Model file for the job. Use its own axes, mm. Give positions to 0.01 mm unless a question says otherwise; leave off trailing zeros. Write each loop counter-clockwise with the first axis right and the second up, starting at its lowest first coordinate (ties: lowest second). Pieces come first, ordered by that corner, then holes. Notation, with made-up numbers: (68, -10.5) - (72, -10.5) arc R5 ccw to (72, -5.5) - close; hole circle Ø4 at (-31, 55). An arc over 180 degrees is marked (long way). Use CSV: the item, a comma, the result in double quotes.
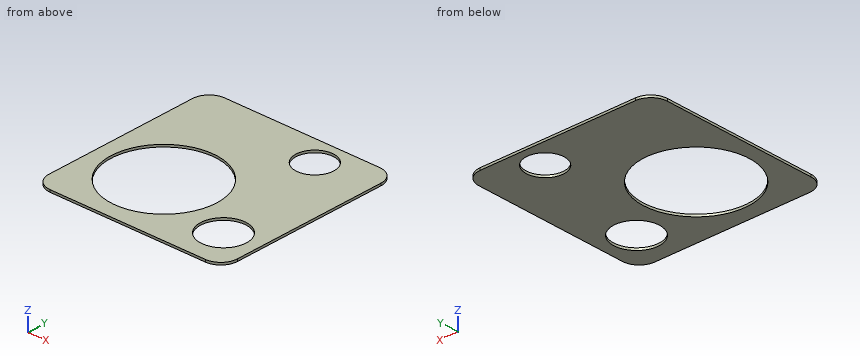
from build123d import *

# Parameters (mm, degrees)
SKETCH1_W           = 500
SKETCH1_H           = 501
BOSS_EXTRUDE1_DEPTH = 6
FILLET1_R           = 44
SKETCH3_R           = 140
CUT_EXTRUDE2_DEPTH  = 7
SKETCH5_R           = 60.5
CUT_EXTRUDE3_DEPTH  = 7
SKETCH6_R           = 50
CUT_EXTRUDE5_DEPTH  = 7


with BuildPart() as part:
    # Sketch1 → Boss-Extrude1 (new body)
    with BuildSketch(Plane.XY):
        with Locations((250, 250.5)):
            Rectangle(SKETCH1_W, SKETCH1_H)
    extrude(amount=BOSS_EXTRUDE1_DEPTH)

    # Fillet1
    fillet1_edges = [part.edges().sort_by_distance(p)[0] for p in [
        (0, 501, 3),
        (500, 501, 3),
        (500, 0, 3),
        (0, 0, 3),
    ]]
    fillet(fillet1_edges, radius=FILLET1_R)

    # Sketch3 → Cut-Extrude2 (cut, through all)
    with BuildSketch(Plane.XY.offset(6)):
        with Locations((178.369044072, 181.034738009)):
            Circle(SKETCH3_R)
    extrude(amount=-CUT_EXTRUDE2_DEPTH, mode=Mode.SUBTRACT)

    # Sketch5 → Cut-Extrude3 (cut, through all)
    with BuildSketch(Plane.XY.offset(6)):
        with Locations((409.103373264, 102.516190165)):
            Circle(SKETCH5_R)
    extrude(amount=-CUT_EXTRUDE3_DEPTH, mode=Mode.SUBTRACT)

    # Sketch6 → Cut-Extrude5 (cut, through all)
    with BuildSketch(Plane.XY.offset(6)):
        with Locations((349.228645131, 430)):
            Circle(SKETCH6_R)
    extrude(amount=-CUT_EXTRUDE5_DEPTH, mode=Mode.SUBTRACT)


solid = part.part
(1) Wall check: probe 1 along X at (y, z) = (63, 0.85); probe 2 along X at (y, z) = (178.5, 1.6); probe 3 along Y at (x, z) = (307.5, 4.4). Give the ranges that are in metal, low to high. Write a range as [from, to].
Checked values:
probe 1,"x = [0, 103.08], [253.65, 363.29], [454.92, 500]"
probe 2,"x = [0, 38.39], [318.35, 500]"
probe 3,"y = [0, 126.95], [235.12, 402.46], [457.54, 501]"
(2) Saw through at A-A, the plane y = 430. List the corners of the cut face in (x, z).
Checked values:
outline,"(0, 0) - (299.23, 0) - (299.23, 6) - (0, 6) - close; (399.23, 0) - (500, 0) - (500, 6) - (399.23, 6) - close"
(3) Saw through at C-C, the plane z = 4.65. List the corners of the cut face in (x, y), then the cut area to 3 significant figures.
Checked values:
outline,"(0, 44) arc R44 ccw to (44, 0) - (456, 0) arc R44 ccw to (500, 44) - (500, 457) arc R44 ccw to (456, 501) - (44, 501) arc R44 ccw to (0, 457) - close; hole circle Ø280 at (178.37, 181.03); hole circle Ø100 at (349.23, 430); hole circle Ø121 at (409.1, 102.52)"
area,"168,000 mm^2"
(4) Saw through at D-D, the plane y = 123. List the corners of the cut face in (x, z), then the cut area to 3 significant figures.
Checked values:
outline,"(0, 0) - (50.96, 0) - (50.96, 6) - (0, 6) - close; (305.77, 0) - (352.18, 0) - (352.18, 6) - (305.77, 6) - close; (466.03, 0) - (500, 0) - (500, 6) - (466.03, 6) - close"
area,"788 mm^2"
(5) Saw through at B-B, the plane x = 99.5. List the corners of the cut face in (y, z), then the cut area to 3 significant figures.
Checked values:
outline,"(0, 0) - (65.36, 0) - (65.36, 6) - (0, 6) - close; (296.71, 0) - (501, 0) - (501, 6) - (296.71, 6) - close"
area,"1,620 mm^2"
